Autodesk Inventor part; units mm, degrees
ref_plane "YZ Plane" through (0, 0, 0) normal (1, 0, 0) x (0, 1, 0)
ref_plane "XZ Plane" through (0, 0, 0) normal (0, 1, 0) x (-1, 0, 0)
ref_plane "XY Plane" through (0, 0, 0) normal (0, 0, 1) x (1, 0, 0)
sketch "Sketch1" plane through (0, 0, 0) normal (0, 1, 0) x (-1, 0, 0)
  line L0 (0, 0) -> (25.4, 0)
  line L1 (25.4, 0) -> (25.4, -50.8)
  line L2 (25.4, -50.8) -> (0, -50.8)
  line L3 (0, -50.8) -> (0, 0)
  line L4 (22.225, -3.175) -> (3.175, -3.175)
  line L5 (3.175, -3.175) -> (3.175, -47.625)
  line L6 (3.175, -47.625) -> (22.225, -47.625)
  line L7 (22.225, -47.625) -> (22.225, -3.175)
  dimension "d0" = 25.4
  dimension "d1" = 50.8
  dimension "d2" = 3.175
extrude "Extrusion1" add sketch "Sketch1" along normal blind 106.553
sketch "Sketch3" plane through (0, 0, 0) normal (1, 0, 0) x (0, 0, -1)
  line L0 (50.8, 0) -> (0, 0)
  line L1 (50.8, 0) -> (50.8, 106.553)
  line L2 (0, 106.553) -> (50.8, 106.553)
  line L3 (0, 0) -> (0, 106.553)
  point P0 (25.4, 68.453)
  dimension "d19" = 38.1
hole "Hole2" at (0, 68.453, -25.4) direction (-1, 0, 0) diameter 28.575 end through all
sketch "Sketch4" plane through (0, 0, 0) normal (0, -1, 0) x (1, 0, 0)
  line L0 (-22.225, -47.625) -> (-22.225, -3.175)
  line L1 (-22.225, -3.175) -> (-3.175, -3.175)
  line L2 (-3.175, -3.175) -> (-3.175, -47.625)
  line L3 (-3.175, -47.625) -> (-22.225, -47.625)
  line L4 (0, 0) -> (-25.4, 0)
  line L5 (-25.4, 0) -> (-25.4, -50.8)
  line L6 (-25.4, -50.8) -> (0, -50.8)
  line L7 (0, -50.8) -> (0, 0)
extrude "Extrusion2" add sketch "Sketch4" along normal blind 254
sketch "Sketch5" plane through (0, 106.553, 0) normal (1, 0, 0) x (0, 0, -1)
  circle A0 centre (25.4, -38.1) radius 14.2875
  line L0 (50.8, 0) -> (50.8, -360.553)
  line L1 (0, 0) -> (50.8, 0)
  line L2 (0, -360.553) -> (0, 0)
  line L3 (50.8, -360.553) -> (0, -360.553)
  line L4 (0, -360.553) -> (23.3209, -360.553)
  line L5 (0, -360.553) -> (50.8, -360.553)
  line L6 (0, -360.553) -> (9.2137, -369.7667)
  line L7 (0, -360.553) -> (9.2137, -360.553)
  line L8 (9.2137, -360.553) -> (9.2137, -369.7667)
  line L9 (9.2137, -369.7667) -> (0, -369.7667)
  line L10 (0, -369.7667) -> (0, -360.553)
  line L11 (0, -369.7667) -> (0, -378.9805)
  line L12 (0, -378.9805) -> (50.8, -328.1805)
  line L13 (50.8, 0) -> (50.8, -360.553)
  line L14 (50.8, -328.1805) -> (0, -328.1805)
  line L15 (0, -328.1805) -> (0, -378.9805)
  line L16 (0, -378.9805) -> (50.8, -378.9805)
  line L17 (50.8, -378.9805) -> (50.8, -328.1805)
  point P0 (0, -106.553)
  dimension "d22" = 13.0302
  dimension "d23" = 45
  dimension "d24" = 45
extrude "Extrusion3" add sketch "Sketch5" against normal blind 25.4 contours L12 L3 L2 L14 | L12 L8 L3 | L8 L6 L3 | L9 L10 L6 | L12 L11 L9
extrude "Extrusion4" cut sketch "Sketch5" against normal blind 25.4 contours L0 L3 L12 | L17 L16 L12 L3
sketch "Sketch6" plane through (0, 106.553, 0) normal (0, 1, 0) x (1, 0, 0)
  line L0 (-22.225, 3.175) -> (-22.225, 47.625)
  line L1 (-3.175, 3.175) -> (-22.225, 3.175)
  line L2 (-3.175, 47.625) -> (-3.175, 3.175)
  line L3 (-22.225, 47.625) -> (-3.175, 47.625)
  point P0 (0, 0)
extrude "Extrusion5" cut sketch "Sketch6" against normal through all
sketch "Sketch7" plane through (0, 106.553, 0) normal (1, 0, 0) x (0, 0, -1)
  line L0 (0, -378.9805) -> (50.8, -328.1805)
  line L1 (50.8, 0) -> (50.8, -328.1805)
  line L2 (0, 0) -> (50.8, 0)
  line L3 (0, -378.9805) -> (0, 0)
  circle A0 centre (25.4, -38.1) radius 14.2875
  point P0 (0, -106.553)
  point P1 (25.4, -114.3)
  dimension "d31" = 76.2
hole "Hole3" at (0, -7.747, -25.4) direction (-1, 0, 0) diameter 28.575 end through all
properties part number "StorageSupport.ver1-1111-2020" material "Aluminum 6061"
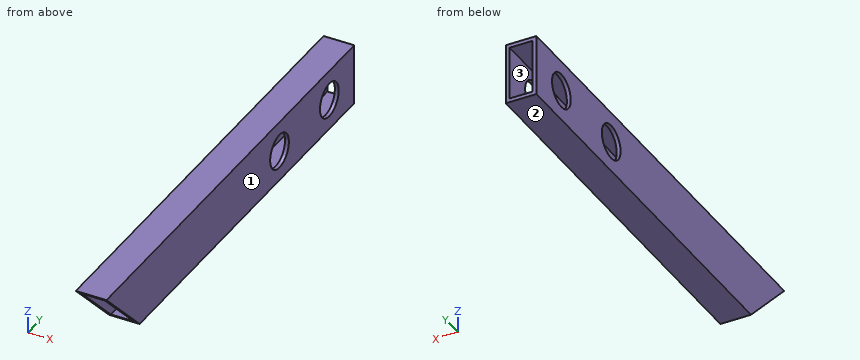
Read the model definition and answer for the solid it produces. Units are mm, in the model's axes. Face numbers are marked on the shaded views. Coordinates: 2 decimals unless noted, no trailing zeros. Loops run counter-clockwise (first coordinate to the right, second up) from the corner with the lowest first, then second, coordinate; pieces in that order, holes last. Notation, with made-up numbers: (85, 1.25) -> (136, 1.25) arc R15 cw to (136, 20.25) -> close; hole circle Ø5 at (0.5, 54.25). An arc over 180 degrees is marked (long way). Answer in a Markdown table with one row per item.
Item 1: A cutting plane is placed at A-A on z = -25.5. Determine the outline of the cut face in (x, y) (1 decimal), plus the area to 3 significant figures.
Returned:
| item | result |
|---|---|
| outline | (-25.4, -246.9) -> (-22.2, -246.9) -> (-22.2, -22) -> (-25.4, -22) -> close; (-25.4, 6.5) -> (-22.2, 6.5) -> (-22.2, 54.2) -> (-25.4, 54.2) -> close; (-25.4, 82.7) -> (-22.2, 82.7) -> (-22.2, 106.6) -> (-25.4, 106.6) -> close; (-3.2, -246.9) -> (0, -246.9) -> (0, -22) -> (-3.2, -22) -> close; (-3.2, 6.5) -> (0, 6.5) -> (0, 54.2) -> (-3.2, 54.2) -> close; (-3.2, 82.7) -> (0, 82.7) -> (0, 106.6) -> (-3.2, 106.6) -> close |
| area | 1,880 mm^2 |
Item 2: Straight lines are drawn through the part: line 1 along Z through (x, y) = (-18, -164.5) (3 decimals); line 2 along X through (y, z) = (-22.5, -5) (3 decimals); line 3 along Y through (x, z) = (-23.75, -33.5). For each, find the intervals that lie inside material, in ascending order. Write a range as [from, to].
Returned:
| item | result |
|---|---|
| line 1 | z = [-50.8, -47.625], [-3.175, 0] |
| line 2 | x = [-25.4, -22.225], [-3.175, 0] |
| line 3 | y = [-238.93, -19.52], [4.02, 56.68], [80.22, 106.55] |
Item 3: A cutting plane is placed at C-C on y = -168. Determine the outline of the cut face in (x, z) (3 decimals), plus the area to 3 significant figures.
Returned:
| item | result |
|---|---|
| outline | (-25.4, -50.8) -> (0, -50.8) -> (0, 0) -> (-25.4, 0) -> close; hole (-22.225, -47.625) -> (-3.175, -47.625) -> (-3.175, -3.175) -> (-22.225, -3.175) -> close |
| area | 444 mm^2 |
Item 4: A cutting plane is placed at D-D on z = -8. Determine the outline of the cut face in (x, y) (1 decimal).
Returned:
| item | result |
|---|---|
| outline | (-25.4, -264.4) -> (-22.2, -264.4) -> (-22.2, 106.6) -> (-25.4, 106.6) -> close; (-3.2, -264.4) -> (0, -264.4) -> (0, 106.6) -> (-3.2, 106.6) -> close |
Item 5: For a pull along Z with two mould halves and no side action, classify the marked faces 1, 2 and 3 as released by +Z, released by -Z, zero draft, split by the parting line, or undercut.
Returned:
| item | result |
|---|---|
| face 1 | zero draft |
| face 2 | released by -Z |
| face 3 | undercut |
Item 6: A cutting plane is placed at B-B on x = -9.75. Determine the outline of the cut face in (y, z) (1 decimal).
Returned:
| item | result |
|---|---|
| outline | (-272.4, 0) -> (-269.3, -3.2) -> (106.6, -3.2) -> (106.6, 0) -> close; (-224.8, -47.6) -> (-221.6, -50.8) -> (106.6, -50.8) -> (106.6, -47.6) -> close |
Item 7: This flat-tipped pin is pushed along its axis until it touches: P1, Ø5.5, axis at x = -14, y = -78.5, coming from the +Z side. Where does it stop, or does it pass through?
Returned:
| item | result |
|---|---|
| P1 | stops at z = 0 |
